```python
from build123d import *

# Parameters (mm, degrees)
F0_W     = 50
F0_H     = 50
F0_R     = 15
F1_DEPTH = 20
F2_R     = 20
F3_DEPTH = 20
F6_R     = 24.99999
F7_R     = 3


# Not quite as in the source:
# - a fillet or chamfer is up to 0.001 mm smaller than in the source, because OpenCascade refuses the exact size


with BuildPart() as f1:
    # F0 (on Top) → F1 (new body)
    with BuildSketch(Plane.XY):
        Rectangle(F0_W, F0_H)
        Circle(F0_R, mode=Mode.SUBTRACT)
    extrude(amount=F1_DEPTH)


with BuildPart() as f3:
    # F2 (on Top) → F3 (new body)
    with BuildSketch(Plane.XY):
        Circle(F2_R)
    extrude(amount=F3_DEPTH)


with BuildPart() as f3_1:
    # F4: moved
    add(f3.part.moved(Location((0, 0, 3))))


with BuildPart() as f1_1:
    add(f1.part)

    # F5: cut F3
    add(f3_1.part, mode=Mode.SUBTRACT)

    # F6 (radius 25 in the source; OpenCascade refuses exactly that, so slightly less here)
    f6_edges = [f1_1.edges().sort_by_distance(p)[0] for p in [
        (-25, 25, 10),
        (-25, -25, 10),
        (25, -25, 10),
        (25, 25, 10),
    ]]
    fillet(f6_edges, radius=F6_R)

    # F7
    f7_edges = [f1_1.edges().sort_by_distance(p)[0] for p in [
        (-17.677672, 17.677672, 0),
        (-17.677672, 17.677672, 20),
    ]]
    fillet(f7_edges, radius=F7_R)


solid = f1_1.part
```
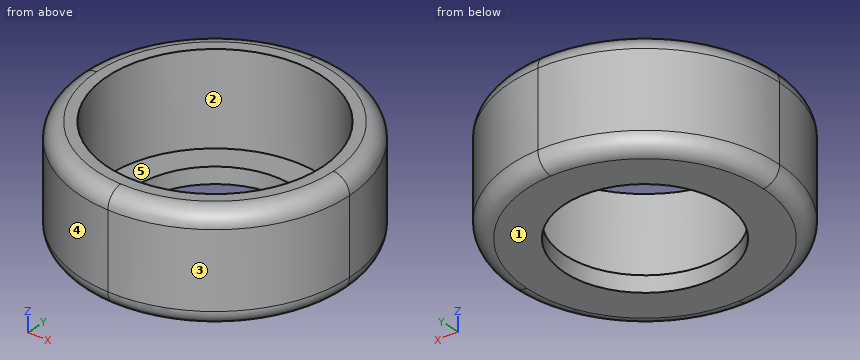
Verification items for the finished model (mm, model axes). Face numbers are marked on the shaded views. A direction names the side the tool comes from. Coordinates: 2 decimals unless noted, no trailing zeros. Answer as a JSON object with one key per item and string values. Group by question number.
(1) Gauge pin test, flat ends, axial feed: pin 1 (10 mm diameter, centred on y = -8, z = 13.5, fed in from +X); pin 2 (4 mm diameter, centred on x = 13.5, y = 0, fed in from +Z); pin 3 (2 mm diameter, centred on y = -20, z = 4, fed in from -X); pin 4 (1 mm diameter, centred on x = 6.5, y = 11, fed in from -Z). Record the tip position at first contact, or that the pin passes through.
(2) Material ranges on line 1 (X direction, y = 0, z = 16.75); line 2 (X direction, y = 14, z = 18); line 3 (Y direction, x = 12, z = 4), recorded low to high.
(3) Tool access check on the marked faces 4 and 5. Record the directions out of +Z, -Z, +X, -X, +Y, -Y that give a thin tool (end or side, any length) a straight path to the whole face; none if there is none.
(4) Release check for a two-part mould opening along Y. For the marked faces 1, 2 and 3 record: +Y half, -Y half, draft (parallel to the pull), parting line (faces both ways), or undercut.
Reply:
{
 "1": {"pin 1": "x = 24.82", "pin 2": "z = 3", "pin 3": "x = -16.25", "pin 4": "through"},
 "2": {"line 1": "-25 to -20, 20 to 25", "line 2": "-20.5 to -14.28, 14.28 to 20.5", "line 3": "-21.93 to -16, 16 to 21.93"},
 "3": {"face 4": "+Z, -Z, -X, -Y", "face 5": "+Z"},
 "4": {"face 1": "draft", "face 2": "undercut", "face 3": "-Y half"}
}
